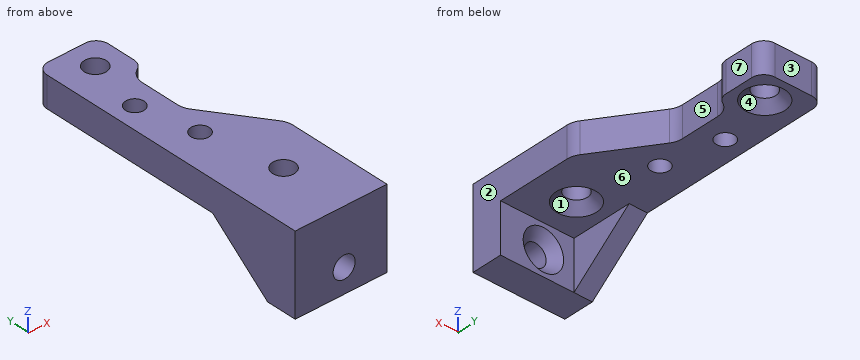
```python
from build123d import *

# Parameters (mm, degrees)
EXTRUDE_1_DEPTH           = 10
EXTRUDE_1_DEPTH_BACK      = 5
EXTRUDE_2_DEPTH           = 5
RIB_4_REACH               = 54.517
SKETCH_2_WALL_W           = 119.839576518
SKETCH_2_WALL_H           = 3
HOLE_WIZARD_1_D           = 3.6
HOLE_WIZARD_1_CSINK_D     = 6.6
HOLE_WIZARD_1_CSINK_ANGLE = 90
MM_TRANSITIONAL_1_D       = 3
FILLET_1_R                = 3
FILLET_2_R                = 2
HOLE_WIZARD_2_D           = 3.6
HOLE_WIZARD_2_CSINK_D     = 6.6
HOLE_WIZARD_2_CSINK_ANGLE = 90


with BuildPart() as part:
    # 草图1 → 凸台-拉伸1 (new, two sides: drawn at the far end of the back side and taken through both)
    with BuildSketch(Plane(origin=(0, 0, 0), x_dir=(0, 0, -1), z_dir=(1, 0, 0)).offset(-EXTRUDE_1_DEPTH_BACK)):
        Polygon((13, 5), (5, 5), (5, 18), (0, 18), (0, 0), (13, 0), align=None)
    extrude(amount=EXTRUDE_1_DEPTH + EXTRUDE_1_DEPTH_BACK)

    # 草图3 → 凸台-拉伸2 (add)
    with BuildSketch(Plane(origin=(-10, 0, -5), x_dir=(-1, 0, 0), z_dir=(0, 0, -1))):
        Polygon((-5, 18), (-5, 47), (-15, 47), (-15, 39), (-12.5, 39), (-12.5, 28.711110051), (-20, 18), align=None)
    extrude(amount=-EXTRUDE_2_DEPTH)

    # 草图2 wall → 筋4 (add, up to next)
    with BuildSketch(Plane(origin=(-5, 10, -9), x_dir=(0, -0.780868809443, -0.624695047554), z_dir=(0, -0.624695047554, 0.780868809443)), mode=Mode.PRIVATE) as rib_4_sk1:
        with Locations((0, 1.5)):
            Rectangle(SKETCH_2_WALL_W, SKETCH_2_WALL_H)
    rib_4_tool1 = extrude(rib_4_sk1.sketch, amount=RIB_4_REACH, mode=Mode.PRIVATE) - part.part
    add(rib_4_tool1.solids().sort_by_distance((-5, 10, -9))[0])

    # 打孔尺寸(%根据十字)槽半沉头木螺钉的类型1 (through all)
    with Locations(Plane(origin=(0, 0, -5), x_dir=(-1, 0, 0), z_dir=(0, 0, -1))):
        with Locations((-3, 11), (-0.608074792, 42.508910889)):
            CounterSinkHole(HOLE_WIZARD_1_D / 2, HOLE_WIZARD_1_CSINK_D / 2, counter_sink_angle=HOLE_WIZARD_1_CSINK_ANGLE)

    # 大小mm Transitional 暗销孔1 (through all)
    with Locations(Plane(origin=(0, 0, -5), x_dir=(-1, 0, 0), z_dir=(0, 0, -1))):
        with Locations((1.5, 33), (-0.608074792, 23.491089111)):
            Hole(MM_TRANSITIONAL_1_D / 2)

    # 圆角1
    # the kernel refuses this fillet: 3 mm, written as the material it adds along each edge
    with BuildSketch(Plane(origin=(2.5, 28.711110051, -5), x_dir=(0.5735764363510514, -0.8191520442889881, 0), z_dir=(0, 0, 1))) as fillet_1_piece_1:
        with BuildLine():
            CenterArc((FILLET_1_R * 0.315298788879, FILLET_1_R), FILLET_1_R, 235, 35)
            Line((-FILLET_1_R * 0.258277647472, FILLET_1_R * 0.180847955711), (0, 0))
            Line((0, 0), (FILLET_1_R * 0.315298788879, 0))
        make_face()
    extrude(amount=5)
    with BuildSketch(Plane(origin=(2.5, 39, -5), x_dir=(0, -1, 0), z_dir=(0, 0, 1))) as fillet_1_piece_2:
        with BuildLine():
            CenterArc((2.958039892, 3), FILLET_1_R, 189.594068227, 80.405931773)
            Line((0, 2.5), (0, 0))
            Line((0, 0), (2.958039892, 0))
        make_face()
    extrude(amount=5)
    # the kernel refuses this fillet: 3 mm, written as the material it takes off along each edge
    with BuildSketch(Plane(origin=(10, 18, -7.364740917), x_dir=(0, -1, 0), z_dir=(0, 0, 1))) as fillet_1_2_piece_1:
        with BuildLine():
            CenterArc((FILLET_1_R * 0.315298788879, -FILLET_1_R), FILLET_1_R, 90, 35)
            Line((-FILLET_1_R * 0.258277647472, -FILLET_1_R * 0.180847955711), (0, 0))
            Line((0, 0), (FILLET_1_R * 0.315298788879, 0))
        make_face()
    extrude(amount=9.729481833, mode=Mode.SUBTRACT)

    # 圆角2
    fillet_2_edges = [part.edges().sort_by_distance(p)[0] for p in [
        (-5, 47, -2.5),
        (5, 47, -2.5),
        (5, 39, -2.5),
    ]]
    fillet(fillet_2_edges, radius=FILLET_2_R)

    # 打孔尺寸(%根据十字)槽半沉头木螺钉的类型2 (through all)
    with Locations(Plane(origin=(0, 5, 0), x_dir=(1, 0, 0), z_dir=(0, 1, 0))):
        with Locations((3, 9)):
            CounterSinkHole(HOLE_WIZARD_2_D / 2, HOLE_WIZARD_2_CSINK_D / 2, counter_sink_angle=HOLE_WIZARD_2_CSINK_ANGLE)


solid = part.part
```
Check sheet for the modelled part. Datum: model origin and axes. Units: mm. Face numbers are marked on the shaded views. A direction names the side the tool comes from. Coordinates: 2 decimals unless noted, no trailing zeros. Write each loop counter-clockwise with the first axis right and the second up, starting at its lowest first coordinate (ties: lowest second). Pieces come first, ordered by that corner, then holes. Notation, with made-up numbers: M -22.75,50 L -14.75,50 A13 cw -14.75,66 Z; hole C 50.5,4.5 d10. An arc over 180 degrees is marked long. Write item = value, one per line. Start each with the question number.
1. Go/stop test with flat-tipped pins: pin 1 (2.5 mm diameter, centred on x = 2, z = -7.5, fed in from +Y); pin 2 (3.5 mm diameter, centred on x = 0.61, y = 23.49, fed in from -Z); pin 3 (2.5 mm diameter, centred on y = 10, z = -8.5, fed in from +X). Record where each tip stops, or that it passes through.
2. Thickness scan on probe 1 along X at (y, z) = (1.15, -9); probe 2 along Y at (x, z) = (-2, -4.75); probe 3 along Z at (x, y) = (6.25, 20). Record the ranges inside material, lowest first.
3. Sectioned sample at C-C (y = 11). Record the cut outline in (x, z), then the cut area to 4 significant figures.
4. Sectioned sample at B-B (z = -4). Record the cut outline in (x, y).
5. Sectioned sample at A-A (y = 33). Record the cut outline in (x, z).
6. Mould release check, pull along Y, two halves, no side actions. Record for the marked faces 1, 2, 3 and 4: pulls with the +Y half, pulls with the -Y half, needs draft (parallel to the pull), parting line crosses it, or undercut.
7. Sectioned sample at D-D (x = 8.25). Record the cut outline in (y, z).
8. Tool access check on the marked faces 5, 6 and 7. Record the directions out of +Z, -Z, +X, -X, +Y, -Y that give a thin tool (end or side, any length) a straight path to the whole face; none if there is none.
The answers:
q1.pin_1 = 4.75
q1.pin_2 = -5
q1.pin_3 = -2
q2.probe_1 = -5 to 1.2, 4.8 to 10
q2.probe_2 = 0 to 31.59, 34.41 to 40.93, 44.09 to 47
q2.probe_3 = -5 to 0
q3.outline = M -5,-8.2 L -2,-8.2 L -2,-5 L -0.3,-5 L 1.2,-3.5 L 1.2,0 L -5,0 Z; M 4.8,-3.5 L 6.3,-5 L 10,-5 L 10,0 L 4.8,0 Z
q3.area = 64.35 mm²
q4.outline = M -5,0 L 10,0 L 10,17.05 A3 ccw 9.46,18.77 L 3.04,27.94 A3 cw 2.5,29.66 L 2.5,36.04 A3 cw 4,38.64 A2 ccw 5,40.37 L 5,45 A2 ccw 3,47 L -3,47 A2 ccw -5,45 Z; hole C -1.5,33 d3; hole C 0.61,42.51 d4.6; hole C 0.61,23.49 d3; hole C 3,11 d4.6
q5.outline = M -5,-5 L -3,-5 L -3,0 L -5,0 Z; M 0,-5 L 2.5,-5 L 2.5,0 L 0,0 Z
q6.face_1 = undercut
q6.face_2 = needs draft
q6.face_3 = pulls with the +Y half
q6.face_4 = undercut
q7.outline = M 0,-13 L 5,-13 L 5,-5 L 20.5,-5 L 20.5,0 L 0,0 Z
q8.face_5 = +Z, -Z, +X
q8.face_6 = -Z, +X, +Y
q8.face_7 = +Z, -Z, +X, +Y
